Answer from the drawing. Dimensions are ordinates in mm from the lowest x, y and z of the part. A direction names the side the tool comes from. Coordinates: 2 decimals unless noted, no trailing zeros. Write each loop counter-clockwise with the first axis right and the second up, starting at its lowest first coordinate (ties: lowest second). Pieces come first, ordered by that corner, then holes. Notation, with made-up numbers: (23.5, -17) -> (82.5, -17) arc R23 cw to (82.5, 22) -> close; hole circle Ø2 at (-4, 78). An arc over 180 degrees is marked (long way). One line per item, written item: value. Start each with the question number.
1. Find section B-B, the plane y = 173. Write down the section's boundary in (x, z).
2. Find section D-D, the plane z = 104. Write down the section's boundary in (x, y), and give its area (3 significant figures).
3. Consider line 1 along Z through (x, y) = (241, 156.5); line 2 along Z through (x, y) = (135, 138.5); line 3 along X through (y, z) = (152, 89) (1 decimal). Determine where each line is inside the solid, lowest interval first.
4. For the marked faces 4, 5 and 6, determine the directions among +Z, -Z, +X, -X, +Y, -Y from which every point of the face is accessible in a straight line to the end or side of a thin tool.
5. Given P1, Ø10, axis at y = 71, z = 66, coming from the +X side; P2, Ø1, axis at x = 250, y = 143, coming from the +Z side; P3, Ø9.5, axis at x = 287, z = 14.5, coming from the -Y side, each flat-ended and moving along its own axis, determine where each tip first touches the part or whether it passes through.
6. Find section A-A, the plane z = 20.5. Write down the section's boundary in (x, y).
7. For a pull along X with two mould halves and no side action, classify the marked faces 1, 2 and 3 as pulls with the +X half, pulls with the -X half, needs draft (parallel to the pull), parting line crosses it, or undercut.
8. Find section C-C, the plane x = 286. Write down the section's boundary in (y, z), and give its area (3 significant figures).
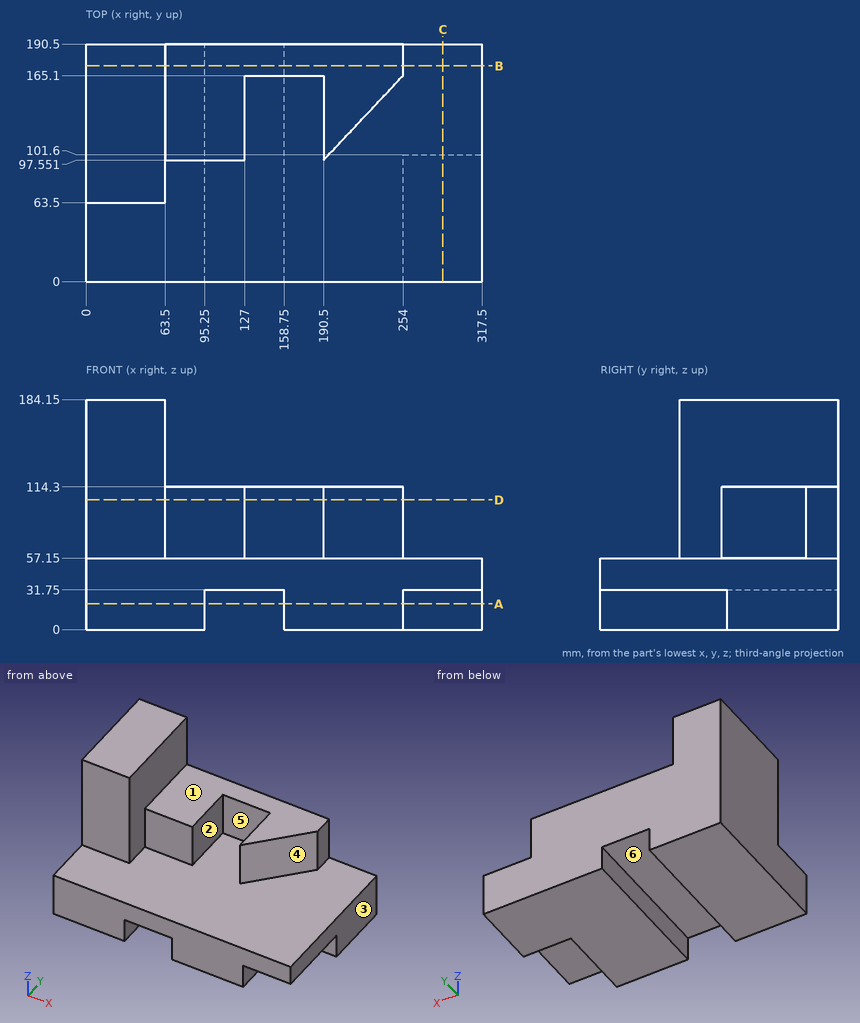
Answer block:
1. outline: (0, 0) -> (95.25, 0) -> (95.25, 31.75) -> (158.75, 31.75) -> (158.75, 0) -> (317.5, 0) -> (317.5, 57.15) -> (254, 57.15) -> (254, 114.3) -> (63.5, 114.3) -> (63.5, 184.15) -> (0, 184.15) -> close
2. outline: (0, 63.5) -> (63.5, 63.5) -> (63.5, 97.55) -> (127, 97.55) -> (127, 165.1) -> (190.5, 165.1) -> (190.5, 97.55) -> (254, 165.1) -> (254, 190.5) -> (0, 190.5) -> close
2. area: 19,300 mm2
3. line 1: z = 0 to 114.3
3. line 2: z = 31.75 to 57.15
3. line 3: x = 0 to 127, 190.5 to 241.7
4. face 4: +Z, +X, -Y
4. face 5: +Z, -Y
4. face 6: -Z, +Y, -Y
5. P1: stops at x = 63.5
5. P2: stops at z = 57.15
5. P3: stops at y = 101.6
6. outline: (0, 0) -> (95.25, 0) -> (95.25, 190.5) -> (0, 190.5) -> close; (158.75, 0) -> (254, 0) -> (254, 101.6) -> (317.5, 101.6) -> (317.5, 190.5) -> (158.75, 190.5) -> close
7. face 1: needs draft
7. face 2: undercut
7. face 3: pulls with the +X half
8. outline: (0, 31.75) -> (101.6, 31.75) -> (101.6, 0) -> (190.5, 0) -> (190.5, 57.15) -> (0, 57.15) -> close
8. area: 7,660 mm2
